```python
from build123d import *

# Parameters (mm, degrees)
F0_W      = 2000
F0_H      = 20
F1_DEPTH  = 30
F2_W      = 10
F2_H      = 10
F3_DEPTH  = 2000
F4_W      = 10
F4_H      = 10
F5_DEPTH  = 2000
F7_START  = -2
F6_W      = 10
F6_H      = 10
F7_DEPTH  = 1996
F8_R      = 3
F9_DEPTH  = 30
F10_R     = 3
F11_DEPTH = 30


with BuildPart() as f1:
    # F0 (on Right) → F1 (new body)
    with BuildSketch(Plane.YZ):
        Rectangle(F0_W, F0_H)
    extrude(amount=F1_DEPTH)

    # F2 (on face) → F3 (join)
    with BuildSketch(Plane.XZ.offset(1000)):
        with Locations((5, 15)):
            Rectangle(F2_W, F2_H)
    extrude(amount=-F3_DEPTH)

    # F4 (on face) → F5 (join)
    with BuildSketch(Plane.XZ.offset(1000)):
        with Locations((25, 15)):
            Rectangle(F4_W, F4_H)
    extrude(amount=-F5_DEPTH)

    # F6 (on face) → F7 (join)
    with BuildSketch(Plane.XZ.offset(1000).offset(F7_START)):
        with Locations((15, -15)):
            Rectangle(F6_W, F6_H)
    extrude(amount=-F7_DEPTH)

    # F8 (on face) → F9 (join)
    with BuildSketch(Plane.XZ.offset(1000)):
        with Locations((15, 0)):
            Circle(F8_R)
    extrude(amount=F9_DEPTH)

    # F10 (on face) → F11 (join)
    with BuildSketch(Plane(origin=(0, 1000, 0), x_dir=(-1, 0, 0), z_dir=(0, 1, 0))):
        with Locations((-15, 0)):
            Circle(F10_R)
    extrude(amount=F11_DEPTH)


solid = f1.part
```
Can you work these out from the model? Positions are in its coordinate system, mm. Give positions to 0.01 mm unless a question says otherwise; leave off trailing zeros. Order: outer loops, then holes, each group sorted by start corner. A loop starts at its lowest first (then second) coordinate and runs counter-clockwise, first axis right, second up. Notation, with made-up numbers: (-8.75, -11.5) - (47.25, -11.5) arc R17 ccw to (47.25, 16.5) - close; hole circle Ø6 at (57, 72.25). An arc over 180 degrees is marked (long way). Use a Markdown table: item, result. Add a question column.
Q1. Please list where these lines run through material, in increasing order: line 1 along X through (y, z) = (-380.5, 16); line 2 along Z through (x, y) = (27.5, -22); line 3 along Z through (x, y) = (16.75, -910).
Q2. If we section it at B-B on x = 4.5: Write out the boundary of the cut face in (y, z).
Q3. I'm going to push flat-ended pins straight in: pin 1 (12 mm diameter, centred on x = 10, z = -9, fed in from -Y); pin 2 (5 mm diameter, centred on x = 15.5, z = -14.5, fed in from +Y); pin 3 (8 mm diameter, centred on x = 15.5, z = -15.5, fed in from -Y). Where does each tip first touch, or does it pass through?
Q4. If we section it at A-A on y = -437: Write out the boundary of the cut face in (x, z).
Answers follow:
| question | item | result |
|---|---|---|
| 1 | line 1 | x = 0 to 10, 20 to 30 |
| 1 | line 2 | z = -10 to 20 |
| 1 | line 3 | z = -20 to 10 |
| 2 | outline | (-1000, -10) - (1000, -10) - (1000, 20) - (-1000, 20) - close |
| 3 | pin 1 | stops at y = -1000 |
| 3 | pin 2 | stops at y = 998 |
| 3 | pin 3 | stops at y = -998 |
| 4 | outline | (0, -10) - (10, -10) - (10, -20) - (20, -20) - (20, -10) - (30, -10) - (30, 20) - (20, 20) - (20, 10) - (10, 10) - (10, 20) - (0, 20) - close |
